The listing builds one solid part. Answer for the finished solid, in the listing's coordinates (mm). Face numbers are marked on the shaded views. A direction names the side the tool comes from. Give positions to 0.01 mm unless a question says otherwise; leave off trailing zeros. Write each loop counter-clockwise with the first axis right and the second up, starting at its lowest first coordinate (ties: lowest second). Pieces come first, ordered by that corner, then holes. Notation, with made-up numbers: M -11,-34.5 L 48,-34.5 A29 cw 48,-13.5 Z; hole C -2,22.25 d8. An arc over 180 degrees is marked long. Answer as a JSON object with one key per item and string values.
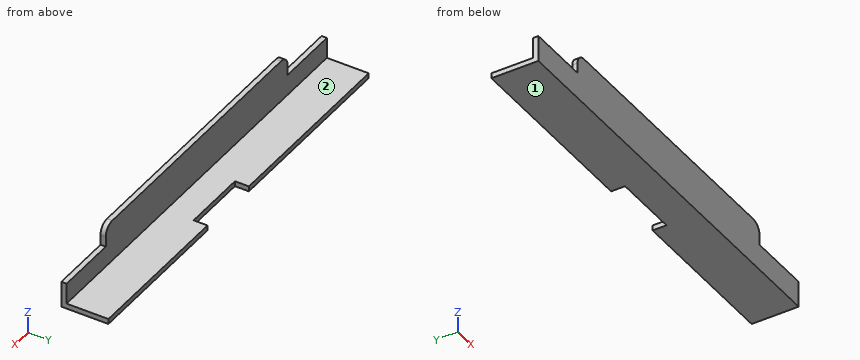
```python
from build123d import *

# Parameters (mm, degrees)
SKETCH2_W           = 239
SKETCH2_H           = 27
BOSS_EXTRUDE1_DEPTH = 3
SKETCH3_W           = 239
SKETCH3_H           = 3
BOSS_EXTRUDE2_DEPTH = 12
BOSS_EXTRUDE4_DEPTH = 3
SKETCH5_W           = 38
SKETCH5_H           = 8
CUT_EXTRUDE1_DEPTH  = 3


with BuildPart() as part:
    # Sketch2 → Boss-Extrude1 (new body)
    with BuildSketch(Plane.XY):
        with Locations((-119.5, -13.5)):
            Rectangle(SKETCH2_W, SKETCH2_H)
    extrude(amount=BOSS_EXTRUDE1_DEPTH)

    # Sketch3 → Boss-Extrude2 (add)
    with BuildSketch(Plane.XY.offset(3)):
        with Locations((-119.5, -25.5)):
            Rectangle(SKETCH3_W, SKETCH3_H)
    extrude(amount=BOSS_EXTRUDE2_DEPTH)

    # Sketch4 → Boss-Extrude4 (add)
    with BuildSketch(Plane(origin=(0, -24, 0), x_dir=(1, 0, 0), z_dir=(0, 1, 0))):
        with BuildLine():
            Line((-203, -15), (-36, -15))
            Line((-36, -15), (-36, -21))
            ThreePointArc((-36, -21), (-37.757359313, -25.242640687), (-42, -27))
            Line((-42, -27), (-197, -27))
            ThreePointArc((-197, -27), (-201.242640687, -25.242640687), (-203, -21))
            Line((-203, -21), (-203, -15))
        make_face()
    extrude(amount=-BOSS_EXTRUDE4_DEPTH)

    # Sketch5 → Cut-Extrude1 (cut)
    with BuildSketch(Plane(origin=(0, 0, 0), x_dir=(-1, 0, 0), z_dir=(0, 0, -1))):
        with Locations((110, -4)):
            Rectangle(SKETCH5_W, SKETCH5_H)
    extrude(amount=-CUT_EXTRUDE1_DEPTH, mode=Mode.SUBTRACT)


solid = part.part
```
1. For the marked faces 1 and 2, determine the directions among +Z, -Z, +X, -X, +Y, -Y from which every point of the face is accessible in a straight line to the end or side of a thin tool.
Verdict:
{"face 1": "-Z, +X, -X, +Y, -Y", "face 2": "+Z, +X, -X, +Y"}
2. A cutting plane is placed at C-C, the plane y = -17.25. Give the vertices of the cut face in (x, z), plus the area to 3 significant figures.
Verdict:
{"outline": "M -239,0 L 0,0 L 0,3 L -239,3 Z", "area": "717 mm2"}
3. A cutting plane is placed at D-D, the plane z = 18.75. Give the vertices of the cut face in (x, y), plus the area to 3 significant figures.
Verdict:
{"outline": "M -203,-27 L -36,-27 L -36,-24 L -203,-24 Z", "area": "501 mm2"}
4. A cutting plane is placed at A-A, the plane y = -5. Give the vertices of the cut face in (x, z).
Verdict:
{"outline": "M -239,0 L -129,0 L -129,3 L -239,3 Z; M -91,0 L 0,0 L 0,3 L -91,3 Z"}
5. A cutting plane is placed at B-B, the plane x = -76. Give the vertices of the cut face in (y, z), plus the area to 3 significant figures.
Verdict:
{"outline": "M -27,0 L 0,0 L 0,3 L -24,3 L -24,27 L -27,27 Z", "area": "153 mm2"}
6. Flat-ended cylindrical pins translate along their axes: pin 1 (12 mm diameter, centred on x = -66, z = 11.5, fed in from +Y); pin 2 (1.5 mm diameter, centred on x = -229, y = -25, fed in from +Z); pin 3 (4 mm diameter, centred on x = -210.5, z = 18.5, fed in from +Y); pin 4 (1.5 mm diameter, centred on y = -25, z = 18.5, fed in from -X). Find the tip coordinate at first contact, or state that the pin passes through.
Verdict:
{"pin 1": "stops at y = -24", "pin 2": "stops at z = 15", "pin 3": "passes through", "pin 4": "stops at x = -203"}
7. Consider line 1 along Z through (x, y) = (-144.5, -23.5); line 2 along Y through (x, z) = (-111, 16). Determine where each line is inside the solid, lowest interval first.
Verdict:
{"line 1": "z = 0 to 3", "line 2": "y = -27 to -24"}
